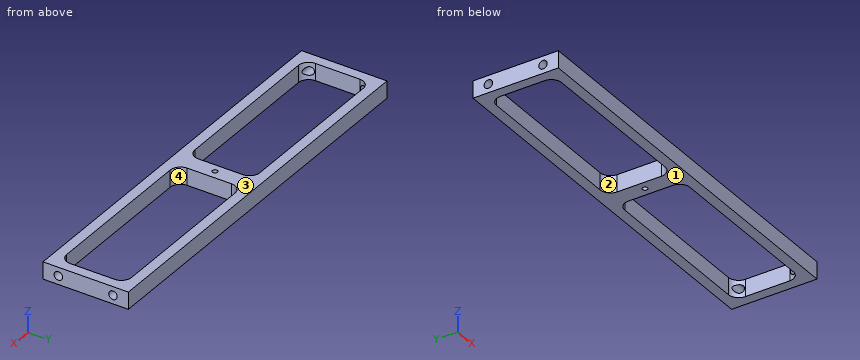
```python
from build123d import *

# Parameters (mm, degrees)
SKETCH_1_W          = 5
SKETCH_1_H          = 38
EXTRUDE_1_DEPTH     = 10
FILLET_1_R          = 6
SKETCH_8_R          = 2.5
CUT_EXTRUDE_4_DEPTH = 91
CUT_EXTRUDE_START   = -91
SKETCH_10_R         = 2.5
CUT_EXTRUDE_5_DEPTH = 91
SKETCH_15_R         = 1.5
CUT_EXTRUDE_9_DEPTH = 10


with BuildPart() as part:
    # 草图1 → 凸台-拉伸1 (new body)
    with BuildSketch(Plane.XY):
        Polygon((6, 6), (6, 44), (110, 44), (115, 44), (115, 50), (0, 50), (0, 0), (115, 0), (115, 6), (110, 6), align=None)
        with Locations((117.5, 25)):
            Rectangle(SKETCH_1_W, SKETCH_1_H)
        with Locations((112.5, 25)):
            Rectangle(SKETCH_1_W, SKETCH_1_H)
        Polygon((115, 50), (115, 44), (120, 44), (224, 44), (224, 6), (120, 6), (115, 6), (115, 0), (230, 0), (230, 50), align=None)
    extrude(amount=EXTRUDE_1_DEPTH)

    # 圆角1
    fillet_1_edges = [part.edges().sort_by_distance(p)[0] for p in [
        (110, 44, 5),
        (6, 44, 5),
        (6, 6, 5),
        (110, 6, 5),
        (120, 6, 5),
        (224, 6, 5),
        (224, 44, 5),
        (120, 44, 5),
    ]]
    fillet(fillet_1_edges, radius=FILLET_1_R)

    # 草图8 → 切除-拉伸4 (cut)
    with BuildSketch(Plane.ZY):
        with Locations((5, 41)):
            Circle(SKETCH_8_R)
        with Locations((5, 9)):
            Circle(SKETCH_8_R)
    extrude(amount=-CUT_EXTRUDE_4_DEPTH, mode=Mode.SUBTRACT)

    # 草图10 → 切除-拉伸5 (cut)
    with BuildSketch(Plane(origin=(230, 0, 0), x_dir=(0, 0, -1), z_dir=(1, 0, 0)).offset(CUT_EXTRUDE_START)):
        with Locations(Location((-5, 41, 0), (0, 0, 180))):
            Circle(SKETCH_10_R)
        with Locations(Location((-5, 9, 0), (0, 0, 180))):
            Circle(SKETCH_10_R)
    extrude(amount=CUT_EXTRUDE_5_DEPTH, mode=Mode.SUBTRACT)

    # 草图15 → 切除-拉伸9 (cut)
    with BuildSketch(Plane.XY.offset(10)):
        with Locations((115, 25)):
            Circle(SKETCH_15_R)
    extrude(amount=-CUT_EXTRUDE_9_DEPTH, mode=Mode.SUBTRACT)


solid = part.part
```
Geometry: final body of the model. Coordinates: model frame, mm. Face numbers are marked on the shaded views. A direction names the side the tool comes from. Give positions to 0.01 mm unless a question says otherwise; leave off trailing zeros. Order: outer loops, then holes, each group sorted by start corner. A loop starts at its lowest first (then second) coordinate and runs counter-clockwise, first axis right, second up. Notation, with made-up numbers: M 80,19 L 91,19 A21 ccw 91,54 Z; hole C 59,14 d2. An arc over 180 degrees is marked long. Answer as CSV lines item,"result". Start each with the question number.
1) Cut plane C-C (z = 5). State how many separate pieces and enclosed holes the cut face has, then the cut area to 3 significant figures.
2) Cut plane A-A (x = 169). Output: boundary loops of the cut face in (y, z), then the cut area to 3 significant figures.
3) First-contact query: P1, Ø4, axis at y = 41, z = 5, coming from the -X side; P2, Ø4, axis at y = 41, z = 5, coming from the +X side. Flat tips, straight axial feed; report the tip coordinate or a pass-through.
4) Cut plane B-B (y = 19). Output: boundary loops of the cut face in (x, z), then the cut area to 3 significant figures.
5) Mould query, pull axis Y, two halves, no side actions, for the marked faces 3 and 4. Classes: +Y half, -Y half, draft (parallel to the pull), parting line (faces both ways), or undercut.
6) Set-up query: the marked faces 1 and 2. Return all of +Z, -Z, +X, -X, +Y, -Y with unobstructed straight access to the full face (end or side cutting, diameter ignored); none if empty.
7) Line query: line 1 (Y direction, x = 3.25, z = 5); line 2 (X direction, y = 32, z = 9.5); line 3 (Y direction, x = 16, z = 5.5). Output: solid intervals per line, ascending. Write a range as from..to.
8) Cut plane D-D (y = 9). Output: boundary loops of the cut face in (x, z), then the cut area to 3 significant figures.
Findings below:
1,separate pieces,"3"
1,enclosed holes,"1"
1,area,"3,510 mm²"
2,outline,"M 0,0 L 6,0 L 6,10 L 0,10 Z; M 44,0 L 50,0 L 50,10 L 44,10 Z"
2,area,"120 mm²"
3,P1,"stops at x = 107.32"
3,P2,"stops at x = 122.68"
4,outline,"M 0,0 L 6,0 L 6,10 L 0,10 Z; M 110,0 L 120,0 L 120,10 L 110,10 Z; M 224,0 L 230,0 L 230,10 L 224,10 Z"
4,area,"220 mm²"
5,face 3,"draft"
5,face 4,"undercut"
6,face 1,"-Z, +X, -X, +Y, -Y"
6,face 2,"+Z, -Z"
7,line 1,"y = 0..6.5, 11.5..38.5, 43.5..50"
7,line 2,"x = 0..6, 110..120, 224..230"
7,line 3,"y = 0..6, 44..50"
8,outline,"M 0,0 L 6.8,0 L 6.8,2.5 L 0,2.5 Z; M 0,7.5 L 6.8,7.5 L 6.8,10 L 0,10 Z; M 109.2,0 L 120.8,0 L 120.8,10 L 109.2,10 Z; M 223.2,0 L 230,0 L 230,2.5 L 223.2,2.5 Z; M 223.2,7.5 L 230,7.5 L 230,10 L 223.2,10 Z"
8,area,"184 mm²"
